```python
from build123d import *

# Parameters (mm, degrees)
SKETCH2_R                      = 13.5
BOSS_EXTRUDE1_DEPTH            = 10
SKETCH3_R                      = 4
BOSS_EXTRUDE2_DEPTH            = 40
CBORE_FOR_M3_SHCS1_D           = 3.2
CBORE_FOR_M3_SHCS1_CBORE_D     = 6.5
CBORE_FOR_M3_SHCS1_CBORE_DEPTH = 5
SKETCH10_R                     = 2.25
CUT_EXTRUDE3_DEPTH             = 7
CHAMFER1_SIZE                  = 0.25
CHAMFER2_SIZE                  = 1


with BuildPart() as part:
    # Sketch2 → Boss-Extrude1 (new body)
    with BuildSketch(Plane(origin=(0, 0, 0), x_dir=(1, 0, 0), z_dir=(0, 1, 0))):
        with Locations(Location((0, 0, 0), (0, 0, 270))):
            Circle(SKETCH2_R)
    extrude(amount=BOSS_EXTRUDE1_DEPTH)

    # Sketch3 → Boss-Extrude2 (add)
    with BuildSketch(Plane(origin=(0, 0, 0), x_dir=(1, 0, 0), z_dir=(0, 1, 0))):
        with Locations(Location((0, 0, 0), (0, 0, 270))):
            Circle(SKETCH3_R)
    extrude(amount=BOSS_EXTRUDE2_DEPTH)

    # CBORE for M3 SHCS1 (through all)
    with Locations(Plane(origin=(0, 10, 0), x_dir=(1, 0, 0), z_dir=(0, 1, 0))):
        with Locations((-9, 0), (9, 0), (0, 9), (0, -9)):
            CounterBoreHole(CBORE_FOR_M3_SHCS1_D / 2, CBORE_FOR_M3_SHCS1_CBORE_D / 2, CBORE_FOR_M3_SHCS1_CBORE_DEPTH)

    # Sketch10 → Cut-Extrude3 (cut)
    with BuildSketch(Plane(origin=(0, 0, 0), x_dir=(1, 0, 0), z_dir=(0, 1, 0))):
        with Locations(Location((0, 0, 0), (0, 0, 270))):
            Circle(SKETCH10_R)
    extrude(amount=CUT_EXTRUDE3_DEPTH, mode=Mode.SUBTRACT)

    # Chamfer1
    chamfer1_edges = [part.edges().sort_by_distance(p)[0] for p in [
        (-3.25, 10, 9),
        (0, 0, -13.5),
        (1.6, 0, 9),
        (5.75, 10, 0),
        (10.6, 0, 0),
        (-3.25, 10, -9),
        (1.6, 0, -9),
        (-12.25, 10, 0),
        (-7.4, 0, 0),
        (0, 10, -13.5),
        (0, 0, -2.25),
        (0, 10, -4),
    ]]
    chamfer(chamfer1_edges, length=CHAMFER1_SIZE)

    # Chamfer2
    chamfer2_edges = [part.edges().sort_by_distance(p)[0] for p in [
        (0, 40, -4),
    ]]
    chamfer(chamfer2_edges, length=CHAMFER2_SIZE)


solid = part.part
```
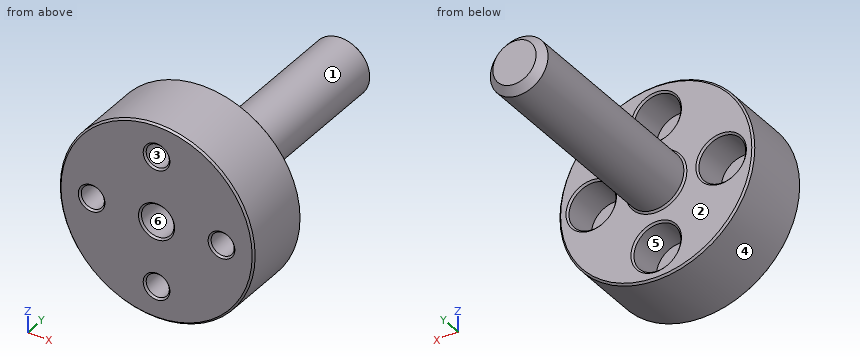
Geometry check sheet. Reference: the model listing, model coordinates, mm. Face numbers are marked on the shaded views. A direction names the side the tool comes from. Coordinates: 2 decimals unless noted, no trailing zeros. Order: outer loops, then holes, each group sorted by start corner. A loop starts at its lowest first (then second) coordinate and runs counter-clockwise, first axis right, second up.
Item 1: Tool access check on the marked faces 4, 5 and 6. Record the directions out of +Z, -Z, +X, -X, +Y, -Y that give a thin tool (end or side, any length) a straight path to the whole face; none if there is none.
Item 2: Depth check by flat-ended pin: pin 1 (3.5 mm diameter, centred on x = 0, z = 9, fed in from +Y); pin 2 (8 mm diameter, centred on x = 4.5, y = 20, fed in from -Z); pin 3 (10 mm diameter, centred on y = 23, z = -1.5, fed in from +X). Enter the tip coordinate at first touch or a pass-through.
Item 3: Section check B-B (z = 0). Count the separate pieces of the cut face and the enclosed holes in it, plus the area to 3 significant figures.
Item 4: Section check D-D (y = 35). Enter the section's corners in (x, z), plus the area to 3 significant figures.
Item 5: Scan lines: line 1 along X through (y, z) = (1.95, 0); line 2 along X through (y, z) = (6.8, 0); line 3 along Y through (x, z) = (6.5, 7.75). Record each from-to range of solid material in increasing order.
Item 6: Section check A-A (y = 8.5). Enter the section's corners in (x, z), plus the area to 3 significant figures.
Item 7: Mould release check, pull along Z, two halves, no side actions. Record for the marked faces 1, 2 and 3: released by +Z, released by -Z, zero draft, split by the parting line, or undercut.
Check sheet entries:
1. face 4: +Y, -Y
1. face 5: +Y
1. face 6: -Y
2. pin 1: stops at y = 5
2. pin 2: stops at z = -3.97
2. pin 3: stops at x = 4
3. separate pieces: 3
3. enclosed holes: 0
3. area: 380 mm2
4. outline: circle Ø8 at (0, 0)
4. area: 50.3 mm2
5. line 1: x = -13.5 to -10.6, -7.4 to -2.25, 2.25 to 7.4, 10.6 to 13.5
5. line 2: x = -13.5 to -12.25, -5.75 to -2.25, 2.25 to 5.75, 12.25 to 13.5
5. line 3: y = 0 to 10
6. outline: circle Ø27 at (0, 0); hole circle Ø6.5 at (-9, 0); hole circle Ø6.5 at (0, -9); hole circle Ø6.5 at (0, 9); hole circle Ø6.5 at (9, 0)
6. area: 440 mm2
7. face 1: split by the parting line
7. face 2: zero draft
7. face 3: undercut
